```python
from build123d import *

# Parameters (mm, degrees)
SKETCH1_W           = 205
SKETCH1_H           = 147
BOSS_EXTRUDE1_DEPTH = 12
SKETCH2_W           = 201.5
SKETCH2_H           = 143.5
CUT_EXTRUDE1_DEPTH  = 9
CUT_EXTRUDE2_DEPTH  = 4
CHAMFER1_SIZE       = 2
FILLET1_R           = 2
SKETCH4_W           = 14
SKETCH4_H           = 5
SKETCH4_W_2         = 20
SKETCH4_H_2         = 4
SKETCH4_W_3         = 7
SKETCH4_W_4         = 20.5
CUT_EXTRUDE3_DEPTH  = 10
SKETCH5_W           = 10
SKETCH5_H           = 10
BOSS_EXTRUDE2_DEPTH = 2
SKETCH6_R           = 1.25
CUT_EXTRUDE4_DEPTH  = 3


with BuildPart() as part:
    # Sketch1 → Boss-Extrude1 (new body)
    with BuildSketch(Plane(origin=(0, 0, 0), x_dir=(1, 0, 0), z_dir=(0, 1, 0))):
        Rectangle(SKETCH1_W, SKETCH1_H)
    extrude(amount=BOSS_EXTRUDE1_DEPTH)

    # Sketch2 → Cut-Extrude1 (cut)
    with BuildSketch(Plane(origin=(0, 12, 0), x_dir=(1, 0, 0), z_dir=(0, 1, 0))):
        Rectangle(SKETCH2_W, SKETCH2_H)
    extrude(amount=-CUT_EXTRUDE1_DEPTH, mode=Mode.SUBTRACT)

    # Sketch3 → Cut-Extrude2 (cut, through all)
    with BuildSketch(Plane(origin=(0, 3, 0), x_dir=(1, 0, 0), z_dir=(0, 1, 0))):
        Polygon((23.033460859, 0.25), (19.39173043, 6.557662131), (12.10826957, 6.557662131), (8.466539141, 0.25), (12.10826957, -6.057662131), (19.39173043, -6.057662131), align=None)
        Polygon((47.75, 18.125), (41.75, 28.517304845), (29.75, 28.517304845), (23.75, 18.125), (29.75, 7.732695155), (41.75, 7.732695155), align=None)
        Polygon((47.75, -18.12), (41.75, -7.727695155), (29.75, -7.727695155), (23.75, -18.12), (29.75, -28.512304845), (41.75, -28.512304845), align=None)
        Polygon((79.75, 0.25), (72.75, 12.374355653), (58.75, 12.374355653), (51.75, 0.25), (58.75, -11.874355653), (72.75, -11.874355653), align=None)
        Polygon((79.75, -36), (72.75, -23.875644347), (58.75, -23.875644347), (51.75, -36), (58.75, -48.124355653), (72.75, -48.124355653), align=None)
        Polygon((79.75, 36), (72.75, 48.124355653), (58.75, 48.124355653), (51.75, 36), (58.75, 23.875644347), (72.75, 23.875644347), align=None)
        Polygon((-19.39173043, -6.057662131), (-23.033460859, 0.25), (-19.39173043, 6.557662131), (-12.10826957, 6.557662131), (-8.466539141, 0.25), (-12.10826957, -6.057662131), align=None)
        Polygon((-72.75, 23.875644347), (-79.75, 36), (-72.75, 48.124355653), (-58.75, 48.124355653), (-51.75, 36), (-58.75, 23.875644347), align=None)
        Polygon((-72.75, -48.124355653), (-79.75, -36), (-72.75, -23.875644347), (-58.75, -23.875644347), (-51.75, -36), (-58.75, -48.124355653), align=None)
        Polygon((-72.75, -11.874355653), (-79.75, 0.25), (-72.75, 12.374355653), (-58.75, 12.374355653), (-51.75, 0.25), (-58.75, -11.874355653), align=None)
        Polygon((-41.75, -28.512304845), (-47.75, -18.12), (-41.75, -7.727695155), (-29.75, -7.727695155), (-23.75, -18.12), (-29.75, -28.512304845), align=None)
        Polygon((-41.75, 7.732695155), (-47.75, 18.125), (-41.75, 28.517304845), (-29.75, 28.517304845), (-23.75, 18.125), (-29.75, 7.732695155), align=None)
    extrude(amount=-CUT_EXTRUDE2_DEPTH, mode=Mode.SUBTRACT)

    # Chamfer1
    chamfer1_edges = [part.edges().sort_by_distance(p)[0] for p in [
        (-100.75, 3, 0),
        (0, 3, -71.75),
        (100.75, 3, 0),
        (0, 3, 71.75),
        (0, 0, -73.5),
        (102.5, 0, 0),
        (0, 0, 73.5),
        (-102.5, 0, 0),
    ]]
    chamfer(chamfer1_edges, length=CHAMFER1_SIZE)

    # Fillet1
    fillet1_edges = [part.edges().sort_by_distance(p)[0] for p in [
        (100.75, 8.5, -71.75),
        (100.75, 8.5, 71.75),
        (-100.75, 8.5, 71.75),
        (-100.75, 8.5, -71.75),
        (-102.5, 7, -73.5),
        (102.5, 7, -73.5),
        (102.5, 7, 73.5),
        (-102.5, 7, 73.5),
    ]]
    fillet(fillet1_edges, radius=FILLET1_R)

    # Sketch4 → Cut-Extrude3 (cut)
    with BuildSketch(Plane(origin=(102.5, 0, 0), x_dir=(0, 0, -1), z_dir=(1, 0, 0))):
        with Locations((-39, 9.5)):
            Rectangle(SKETCH4_W, SKETCH4_H)
        with Locations((-9, 10)):
            Rectangle(SKETCH4_W_2, SKETCH4_H_2)
        with Locations((15.5, 10)):
            Rectangle(SKETCH4_W_3, SKETCH4_H_2)
        with Locations((54.75, 10)):
            Rectangle(SKETCH4_W_4, SKETCH4_H_2)
    extrude(amount=-CUT_EXTRUDE3_DEPTH, mode=Mode.SUBTRACT)

    # Sketch5 → Boss-Extrude2 (add)
    with BuildSketch(Plane(origin=(0, 3, 0), x_dir=(1, 0, 0), z_dir=(0, 1, 0))):
        with Locations((-93.75, 64.75)):
            Rectangle(SKETCH5_W, SKETCH5_H)
        with Locations((-93.75, -64.75)):
            Rectangle(SKETCH5_W, SKETCH5_H)
        with Locations((93.75, -64.75)):
            Rectangle(SKETCH5_W, SKETCH5_H)
        with Locations((93.75, 6.796682995)):
            Rectangle(SKETCH5_W, SKETCH5_H)
    extrude(amount=BOSS_EXTRUDE2_DEPTH)

    # Sketch6 → Cut-Extrude4 (cut)
    with BuildSketch(Plane(origin=(0, 5, 0), x_dir=(1, 0, 0), z_dir=(0, 1, 0))):
        with Locations((-94, -65.2)):
            Circle(SKETCH6_R)
        with Locations((-94, 65)):
            Circle(SKETCH6_R)
        with Locations((94.5, 6.5)):
            Circle(SKETCH6_R)
        with Locations((94.5, -65.2)):
            Circle(SKETCH6_R)
    extrude(amount=-CUT_EXTRUDE4_DEPTH, mode=Mode.SUBTRACT)


solid = part.part
```
Design review of the part built by this model. Coordinates are the model's own, in mm. A direction names the side the tool comes from. Coordinates: 2 decimals unless noted, no trailing zeros. Write each loop counter-clockwise with the first axis right and the second up, starting at its lowest first coordinate (ties: lowest second). Pieces come first, ordered by that corner, then holes.
1) To check wall thickness, follow L1, parallel to Z at x = 94.5, y = 2.75; L2, parallel to Z at x = -36.5, y = 11.5; L3, parallel to X at y = 0.75, z = 33. State the ranges of each line that lie inside material, in increasing order.
2) Add section A-A (x = 34.5). Write out the cut boundary in (y, z), plus the area to 3 significant figures.
3) Add section C-C (z = 43). Write out the cut boundary in (x, y), plus the area to 3 significant figures.
4) Machinability: for faces 1 (the flat face through (26.79, 1.52, -23.39)), 2 (the flat face through (93, 5, 65)), 3 (the flat face through (-1, 7, 73.5)), which of the approach directions +Z, -Z, +X, -X, +Y, -Y give a long, thin tool a straight path to every point of the face, cutting with its end or side? Answer none if there is none.
5) Add section D-D (z = 2). Write out the cut boundary in (x, y).
6) Mouldability with a two-part tool opening along X and no side actions: class faces 4 (the flat face through (-1, 0, -1)), 5 (the flat face through (102.5, 6, 1)), 6 (the flat face through (55.201, 1.521, -30.023)) as +X half, -X half, draft (parallel to the pull), parting line (faces both ways), or undercut.
7) Insertion check: pin 1 (4 mm diameter, centred on x = 32, z = 51, fed in from +Y); pin 2 (1.4 mm diameter, centred on x = 102, z = -14, fed in from +Y); pin 3 (0.5 mm diameter, centred on x = 101.5, y = 11, fed in from +Z). Each pin has a flat end and moves straight along its axis. Give the tip position at first contact, or say it passes through.
8) Add section B-B (x = 62). Write out the cut boundary in (y, z), plus the area to 3 significant figures.
Check result:
1. L1: z = -73.5 to -7.75, -5.25 to 63.95, 66.45 to 73.5
1. L2: z = -73.5 to -71.75, 71.75 to 73.5
1. L3: x = -101.25 to -78.02, -53.48 to 53.48, 78.02 to 101.25
2. outline: (0, -71.5) - (2, -73.5) - (12, -73.5) - (12, -71.75) - (5, -71.75) - (3, -69.75) - (3, -28.52) - (0, -28.52) - close; (0, -7.73) - (3, -7.73) - (3, 7.73) - (0, 7.73) - close; (0, 28.51) - (3, 28.51) - (3, 69.75) - (5, 71.75) - (12, 71.75) - (12, 73.5) - (2, 73.5) - (0, 71.5) - close
2. area: 348 mm2
3. outline: (-102.5, 2) - (-100.5, 0) - (-75.71, 0) - (-75.71, 3) - (-98.75, 3) - (-100.75, 5) - (-100.75, 12) - (-102.5, 12) - close; (-55.79, 0) - (55.79, 0) - (55.79, 3) - (-55.79, 3) - close; (75.71, 0) - (100.5, 0) - (102.5, 2) - (102.5, 7) - (100.75, 7) - (100.75, 5) - (98.75, 3) - (75.71, 3) - close
3. area: 518 mm2
4. face 1: +Y, -Y
4. face 2: +Y
4. face 3: +Z, +X, -X, +Y, -Y
5. outline: (-102.5, 2) - (-100.5, 0) - (-78.45, 0) - (-78.45, 3) - (-98.75, 3) - (-100.75, 5) - (-100.75, 12) - (-102.5, 12) - close; (-53.05, 0) - (-21.73, 0) - (-21.73, 3) - (-53.05, 3) - close; (-9.77, 0) - (9.77, 0) - (9.77, 3) - (-9.77, 3) - close; (21.73, 0) - (53.05, 0) - (53.05, 3) - (21.73, 3) - close; (78.45, 0) - (100.5, 0) - (102.5, 2) - (102.5, 8) - (100.75, 8) - (100.75, 5) - (98.75, 3) - (78.45, 3) - close
6. face 4: draft
6. face 5: +X half
6. face 6: undercut
7. pin 1: stops at y = 3
7. pin 2: stops at y = 8
7. pin 3: stops at z = 73.35
8. outline: (0, -71.5) - (2, -73.5) - (12, -73.5) - (12, -71.75) - (5, -71.75) - (3, -69.75) - (3, -48.12) - (0, -48.12) - close; (0, -23.88) - (3, -23.88) - (3, -12.37) - (0, -12.37) - close; (0, 11.87) - (3, 11.87) - (3, 23.88) - (0, 23.88) - close; (0, 48.12) - (3, 48.12) - (3, 69.75) - (5, 71.75) - (12, 71.75) - (12, 73.5) - (2, 73.5) - (0, 71.5) - close
8. area: 254 mm2
